Read the model definition and answer for the solid it produces. Units are mm, in the model's axes. Face numbers are marked on the shaded views. A direction names the side the tool comes from. Give positions to 0.01 mm unless a question says otherwise; leave off trailing zeros. Loops run counter-clockwise (first coordinate to the right, second up) from the corner with the lowest first, then second, coordinate; pieces in that order, holes last. Notation, with made-up numbers: (-15, -14.75) - (26, -14.75) arc R13 cw to (26, -7.75) - close; hole circle Ø2 at (10, -37.5). An arc over 180 degrees is marked (long way). Write each question's results on one line, items separated by ' | '. Start each with the question number.
Q1. Find the intervals of material crossed by line 1 (Y direction, x = -13, z = 18); line 2 (X direction, y = 10, z = 18.75) (3 decimals); line 3 (Y direction, x = 22, z = 11.25), in increasing order. Write a range as from..to.
Q2. The part is cut by section C-C, the plane z = 15.25. Write down the section's boundary in (x, y), plus the area to 3 significant figures.
Q3. Given pin 1 (2 mm diameter, centred on y = -6, z = 13.5, fed in from -X); pin 2 (0.6 mm diameter, centred on y = 10.5, z = 18.5, fed in from +X) (3 decimals); pin 3 (4 mm diameter, centred on x = 16.5, y = -4, fed in from -Z), each flat-ended and moving along its own axis, determine where each tip first touches the part or whether it passes through.
Q4. For the marked faces 1 and 2, determine the directions among +Z, -Z, +X, -X, +Y, -Y from which every point of the face is accessible in a straight line to the end or side of a thin tool.
Q5. The part is cut by section D-D, the plane x = -18.5. Write down the section's boundary in (y, z), plus the area to 3 significant figures.
Q6. The part is cut by section B-B, the plane x = 15. Write down the section's boundary in (y, z), plus the area to 3 significant figures.
Q7. The part is cut by section A-A, the plane y = 1.5. Write down the section's boundary in (x, z) (3 decimals), plus the area to 3 significant figures.
Q8. Determine the mould class of the marked faces 3, 4 and 5 for opening direction Y: +Y half, -Y half, draft (parallel to the pull), parting line (faces both ways), or undercut.
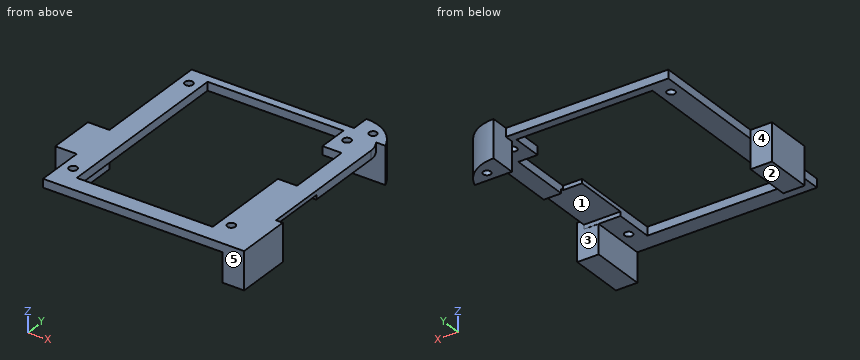
```python
from build123d import *

# Parameters (mm, degrees)
PAD035_DEPTH    = 2
POCKET034_DEPTH = 5
SKETCH080_R     = 0.95
POCKET035_DEPTH = 5
SKETCH081_W     = 5.05
SKETCH081_H     = 13
SKETCH081_H_2   = 11
PAD041_DEPTH    = 8.85
SKETCH082_R     = 0.9
HOLE_DEPTH      = 25
SKETCH086_W     = 8.625
SKETCH086_H     = 13.5
POCKET036_DEPTH = 1


with BuildPart() as part:
    # Sketch071 → Pad035 (new body)
    with BuildSketch(Plane.XY):
        with BuildLine():
            Line((-21.15, 36), (-21.15, -14))
            Line((-21.15, -14), (24.625, -14))
            Line((24.625, -14), (24.625, 31))
            ThreePointArc((24.625, 31), (23.160534, 34.535534), (19.625, 36))
            Line((19.625, 36), (-21.15, 36))
        make_face()
    extrude(amount=-PAD035_DEPTH)

    # Sketch079 (on Face6 of Pad035) → Pocket034 (cut)
    with BuildSketch(Plane.XY):
        Polygon((-16, 34), (-16, -10), (16, -10), (16, 11.95), (20.5, 11.95), (20.5, 26.95), (16, 26.95), (16, 34), align=None)
    extrude(amount=-POCKET034_DEPTH, mode=Mode.SUBTRACT)

    # Sketch080 (on Face4 of Pocket034) → Pocket035 (cut)
    with BuildSketch(Plane.XY):
        with Locations((-18.625, 31.475)):
            Circle(SKETCH080_R)
        with Locations((18.625, 31.475)):
            Circle(SKETCH080_R)
        with Locations((18.625, -7.475)):
            Circle(SKETCH080_R)
        with Locations((-18.625, -7.475)):
            Circle(SKETCH080_R)
    extrude(amount=-POCKET035_DEPTH, mode=Mode.SUBTRACT)

    # Sketch081 (on Face4 of Pocket035) → Pad041 (join)
    with BuildSketch(Plane.XY):
        with Locations((23.675, -7.5)):
            Rectangle(SKETCH081_W, SKETCH081_H)
        with Locations((-23.675, 2.850002)):
            Rectangle(SKETCH081_W, SKETCH081_H_2)
        with BuildLine():
            ThreePointArc((25.850286, 34), (22.447663, 38.458712), (17.1, 40.15))
            Line((17.1, 36), (17.1, 40.15))
            Line((17.1, 36), (17.1, 34))
            Line((17.1, 34), (25.850286, 34))
        make_face()
    extrude(amount=-PAD041_DEPTH)

    # Sketch082 (on Face32 of Pad041) → Hole (cut)
    with BuildSketch(Plane.XY):
        with Locations((21.291797, 36.391807)):
            Circle(SKETCH082_R)
    extrude(amount=-HOLE_DEPTH, mode=Mode.SUBTRACT)

    # Sketch086 (on Face4 of Hole) → Pocket036 (cut)
    with BuildSketch(Plane(origin=(0, 0, -2), x_dir=(1, 0, 0), z_dir=(0, 0, -1))):
        with Locations((20.3125, -5.775)):
            Rectangle(SKETCH086_W, SKETCH086_H)
    extrude(amount=-POCKET036_DEPTH, mode=Mode.SUBTRACT)


with BuildPart() as part_1:
    # Body010 placement: moved
    add(part.part.moved(Location((0, 0, 19.1))))


solid = part_1.part
```
Check sheet entries:
1) line 1: y = -14..-10, 34..36 | line 2: x = -21.15..-16, 16..24.625 | line 3: y = -14..-1, 34..35.84, 36.95..38.75
2) outline: (-26.2, -2.65) - (-21.15, -2.65) - (-21.15, 8.35) - (-26.2, 8.35) - close; (17.1, 34) - (25.85, 34) arc R9.3 ccw to (17.1, 40.15) - close; (21.15, -14) - (26.2, -14) - (26.2, -1) - (21.15, -1) - close; hole circle Ø1.8 at (21.29, 36.39) | area: 158 mm^2
3) pin 1: stops at x = 21.15 | pin 2: stops at x = 24.625 | pin 3: stops at z = 17.1
4) face 1: -Z, +X | face 2: -Z, +X, -X, +Y, -Y
5) outline: (-14, 17.1) - (-8.42, 17.1) - (-8.42, 19.1) - (-14, 19.1) - close; (-6.53, 17.1) - (30.53, 17.1) - (30.53, 19.1) - (-6.53, 19.1) - close; (32.42, 17.1) - (36, 17.1) - (36, 19.1) - (32.42, 19.1) - close | area: 92.5 mm^2
6) outline: (-14, 17.1) - (-10, 17.1) - (-10, 19.1) - (-14, 19.1) - close; (34, 17.1) - (36, 17.1) - (36, 19.1) - (34, 19.1) - close | area: 12.0 mm^2
7) outline: (-26.2, 10.25) - (-21.15, 10.25) - (-21.15, 17.1) - (-16, 17.1) - (-16, 19.1) - (-26.2, 19.1) - close; (16, 18.1) - (24.625, 18.1) - (24.625, 19.1) - (16, 19.1) - close | area: 63.6 mm^2
8) face 3: undercut | face 4: +Y half | face 5: -Y half
